from build123d import *

# Parameters (mm, degrees)
SKETCH_3_W          = 299.999999948
SKETCH_3_H          = 200.00000005
EXTRUDE_1_DEPTH     = 30
FILLET_1_R          = 30
FILLET_2_R          = 30
EXTRUDE_2_DEPTH     = 30
SKETCH_4_R          = 10
CUT_EXTRUDE_1_DEPTH = 30
EXTRUDE_3_DEPTH     = 15


with BuildPart() as part:
    # 草图3 → 凸台-拉伸1 (new body)
    with BuildSketch(Plane(origin=(0, 0, 0), x_dir=(1, 0, 0), z_dir=(0, 1, 0))):
        Rectangle(SKETCH_3_W, SKETCH_3_H)
    extrude(amount=EXTRUDE_1_DEPTH)

    # 圆角1
    fillet_1_edges = [part.edges().sort_by_distance(p)[0] for p in [
        (-149.999999974, 15, 100.000000025),
    ]]
    fillet(fillet_1_edges, radius=FILLET_1_R)

    # 圆角2
    fillet_2_edges = [part.edges().sort_by_distance(p)[0] for p in [
        (149.999999974, 15, 100.000000025),
    ]]
    fillet(fillet_2_edges, radius=FILLET_2_R)

    # 草图5 → 凸台-拉伸2 (add)
    with BuildSketch(Plane(origin=(0, 0, -100.000000025), x_dir=(-1, 0, 0), z_dir=(0, 0, -1))):
        Polygon((-149.999999974, 30), (149.999999974, 30), (40, 130), (-40, 130), align=None)
    extrude(amount=-EXTRUDE_2_DEPTH)

    # 草图4 → 切除-拉伸1 (cut)
    with BuildSketch(Plane(origin=(0, 0, 0), x_dir=(1, 0, 0), z_dir=(0, 1, 0))):
        with Locations(Location((-119.999999974, -70.000000025, 0), (0, 0, 270))):
            Circle(SKETCH_4_R)
        with Locations(Location((119.999999974, -70.000000025, 0), (0, 0, 90))):
            Circle(SKETCH_4_R)
    extrude(amount=CUT_EXTRUDE_1_DEPTH, mode=Mode.SUBTRACT)

    # 草图7 → 凸台-拉伸3 (add, symmetric)
    with BuildSketch(Plane(origin=(0, 0, 0), x_dir=(0, 0, -1), z_dir=(1, 0, 0))):
        Polygon((-70.000000025, 30), (70.000000025, 110), (70.000000025, 30), align=None)
    extrude(amount=EXTRUDE_3_DEPTH, both=True)


solid = part.part
Can you work these out from the model? Positions are in its coordinate system, mm. A direction names the side the tool comes from. Round coordinates to 2 decimals unless told otherwise and drop trailing zeros. Write each loop counter-clockwise with the first axis right and the second up, starting at its lowest first coordinate (ties: lowest second). Pieces come first, ordered by that corner, then holes. Notation, with made-up numbers: (19.25, 32.5) -> (30.25, 32.5) arc R37 cw to (30.25, 69.5) -> close; hole circle Ø11 at (14.5, 47.5). An arc over 180 degrees is marked (long way). One line per question, with ' | ' between items. Start each with the question number.
1) On a 3-axis mill with a long thin cutter (end or side, diameter ignored), from which of +Z, -Z, +X, -X, +Y, -Y can I reach the whole of each face in a straight line? I mean faces 1 (the flat face through (35, 70, -70)), 2 (the flat face through (-15, 53, -32)), 3 (the flat face through (15, 53, -32)). Say none if no direction works.
2) I need wall thicknesses on line 1 (Z direction, x = 120, y = 13.5); line 2 (Y direction, x = -33, z = 26); line 3 (X direction, y = 80, z = -22). Which ranges of each line are inside material? Lowest first, please. Write a range as [from, to].
3) Suppose I cut it at A-A on x = 7. Write out the boundary of the cut face in (y, z).
4) I'm going to push flat-ended pins straight in: P1, Ø6, axis at x = -6, z = -12, coming from the +Y side; P2, Ø2, axis at x = -32, z = -53.5, coming from the +Y side; P3, Ø24, axis at y = 70, z = 22, coming from the -X side. Where does each tip first touch, or does it pass through?
5) Suppose I cut it at D-D on x = 58. Write out the boundary of the cut face in (y, z).
6) If we mould it in two halves opening along Z, with no side actions, what happens to faces 4 (the flat face through (2, 51, -100)), 5 (the flat face through (0.21, 69.44, 0.98)), 6 (the flat face through (94.23, 80.7, -85.21)), 7 (the cylindrical face through (128.872, 14.79, 65.386))? For each: released by +Z, released by -Z, zero draft, split by the parting line, or undercut.
7) Suppose I cut it at B-B on y = 80. Write out the boundary of the cut face in (x, z), then the cut area to 4 significant figures.
8) Suppose I cut it at C-C on z = 28. Write out the boundary of the cut face in (x, y).
Return value:
1) face 1: +Z, +Y | face 2: +Z, -X, +Y | face 3: +Z, +X, +Y
2) line 1: z = [-100, 60], [80, 100] | line 2: y = [0, 30] | line 3: x = [-15, 15]
3) outline: (0, -100) -> (130, -100) -> (130, -70) -> (110, -70) -> (30, 70) -> (30, 100) -> (0, 100) -> close
4) P1: stops at y = 78.57 | P2: stops at y = 30 | P3: stops at x = -15
5) outline: (0, -100) -> (113.64, -100) -> (113.64, -70) -> (30, -70) -> (30, 100) -> (0, 100) -> close
6) face 4: released by -Z | face 5: released by +Z | face 6: zero draft | face 7: undercut
7) outline: (-95, -100) -> (95, -100) -> (95, -70) -> (15, -70) -> (15, -17.5) -> (-15, -17.5) -> (-15, -70) -> (-95, -70) -> close | area: 7,275 mm2
8) outline: (-150, 0) -> (150, 0) -> (150, 30) -> (15, 30) -> (15, 54) -> (-15, 54) -> (-15, 30) -> (-150, 30) -> close
